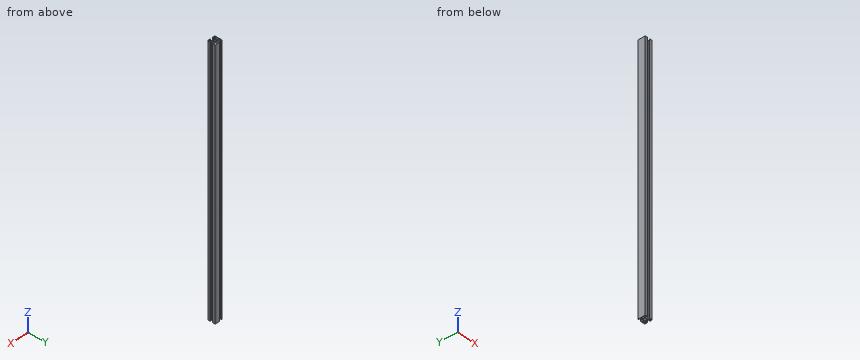
from build123d import *

# Parameters (mm, degrees)
SKETCH_1_R      = 2.25
EXTRUDE_1_DEPTH = 1000


with BuildPart() as part:
    # 草图1 → 拉伸1 (new body)
    with BuildSketch(Plane.XY):
        with BuildLine():
            Line((94.498219996, 123.603787887), (95.498219996, 123.603787887))
            Line((95.498219996, 123.603787887), (95.498219996, 120.604545229))
            Line((95.498219996, 120.604545229), (111.7555793, 120.604545229))
            ThreePointArc((111.7555793, 120.604545229), (112.138262733, 120.680665697), (112.462686082, 120.897438448))
            Line((112.462686082, 120.897438448), (114.705326774, 123.140079141))
            ThreePointArc((114.705326774, 123.140079141), (114.922099526, 123.46450249), (114.998219993, 123.847185922))
            Line((114.998219993, 123.847185922), (114.998219993, 125.604545228))
            ThreePointArc((114.998219993, 125.604545228), (114.705326774, 126.311652009), (113.998219993, 126.604545228))
            Line((113.998219993, 126.604545228), (104.998159012, 126.604545228))
            Line((104.998159012, 126.604545228), (104.998159012, 128.104545228))
            ThreePointArc((104.998159012, 128.104545228), (105.144605621, 128.458098618), (105.498159012, 128.604545228))
            Line((105.498159012, 128.604545228), (120.998159011, 128.604545228))
            ThreePointArc((120.998159011, 128.604545228), (122.412372573, 128.01875879), (122.998159011, 126.604545228))
            Line((122.998159011, 126.604545228), (122.998159011, 118.504545232))
            Line((122.998159011, 118.504545232), (122.198159011, 118.504545232))
            Line((122.198159011, 118.504545232), (122.198159011, 117.704545232))
            Line((122.198159011, 117.704545232), (120.798219991, 117.704545232))
            Line((120.798219991, 117.704545232), (120.798219991, 120.604545232))
            ThreePointArc((120.798219991, 120.604545232), (120.505326773, 121.311652013), (119.798219991, 121.604545232))
            Line((119.798219991, 121.604545232), (117.826647118, 121.604545232))
            ThreePointArc((117.826647118, 121.604545232), (117.443963686, 121.528424765), (117.119540337, 121.311652013))
            Line((117.119540337, 121.311652013), (115.291113212, 119.483224889))
            ThreePointArc((115.291113212, 119.483224889), (115.074340461, 119.15880154), (114.998219993, 118.776118107))
            Line((114.998219993, 118.776118107), (114.998219993, 108.432972357))
            ThreePointArc((114.998219993, 108.432972357), (115.074340461, 108.050288925), (115.291113212, 107.725865576))
            Line((115.291113212, 107.725865576), (117.119540337, 105.897438451))
            ThreePointArc((117.119540337, 105.897438451), (117.443963686, 105.6806657), (117.826647118, 105.604545232))
            Line((117.826647118, 105.604545232), (119.798219991, 105.604545232))
            ThreePointArc((119.798219991, 105.604545232), (120.505326773, 105.897438451), (120.798219991, 106.604545232))
            Line((120.798219991, 106.604545232), (120.798219991, 109.504545225))
            Line((120.798219991, 109.504545225), (122.198159011, 109.504545225))
            Line((122.198159011, 109.504545225), (122.198159011, 108.704545225))
            Line((122.198159011, 108.704545225), (122.998159011, 108.704545225))
            Line((122.998159011, 108.704545225), (122.998159011, 100.60454523))
            ThreePointArc((122.998159011, 100.60454523), (122.412372573, 99.190331667), (120.998159011, 98.60454523))
            Line((120.998159011, 98.60454523), (112.898159016, 98.60454523))
            Line((112.898159016, 98.60454523), (112.898159016, 99.40454523))
            Line((112.898159016, 99.40454523), (112.098159016, 99.40454523))
            Line((112.098159016, 99.40454523), (112.098159016, 100.804545237))
            Line((112.098159016, 100.804545237), (114.998219996, 100.804545237))
            ThreePointArc((114.998219996, 100.804545237), (115.705326777, 101.097438456), (115.998219996, 101.804545237))
            Line((115.998219996, 101.804545237), (115.998219996, 103.77611811))
            ThreePointArc((115.998219996, 103.77611811), (115.922099529, 104.158801543), (115.705326777, 104.483224892))
            Line((115.705326777, 104.483224892), (113.876899653, 106.311652016))
            ThreePointArc((113.876899653, 106.311652016), (113.552476304, 106.528424768), (113.169792871, 106.604545235))
            Line((113.169792871, 106.604545235), (102.826647121, 106.604545235))
            ThreePointArc((102.826647121, 106.604545235), (102.443963688, 106.528424768), (102.11954034, 106.311652016))
            Line((102.11954034, 106.311652016), (100.291113215, 104.483224892))
            ThreePointArc((100.291113215, 104.483224892), (100.074340464, 104.158801543), (99.998219996, 103.77611811))
            Line((99.998219996, 103.77611811), (99.998219996, 101.804545237))
            ThreePointArc((99.998219996, 101.804545237), (100.291113215, 101.097438456), (100.998219996, 100.804545237))
            Line((100.998219996, 100.804545237), (103.898159009, 100.804545237))
            Line((103.898159009, 100.804545237), (103.898159009, 99.40454523))
            Line((103.898159009, 99.40454523), (103.098159009, 99.40454523))
            Line((103.098159009, 99.40454523), (103.098159009, 98.60454523))
            Line((103.098159009, 98.60454523), (94.998159011, 98.60454523))
            ThreePointArc((94.998159011, 98.60454523), (93.583945449, 99.190331667), (92.998159011, 100.60454523))
            Line((92.998159011, 100.60454523), (92.998159011, 126.604545228))
            ThreePointArc((92.998159011, 126.604545228), (93.583945449, 128.01875879), (94.998159011, 128.604545228))
            Line((94.998159011, 128.604545228), (95.498219996, 128.604545228))
            Line((95.498219996, 128.604545228), (95.498219996, 125.603787887))
            Line((95.498219996, 125.603787887), (94.498219996, 125.603787887))
            Line((94.498219996, 125.603787887), (94.498219996, 123.603787887))
        make_face()
        with Locations((119.498219995, 102.104545233)):
            Circle(SKETCH_1_R, mode=Mode.SUBTRACT)
        with BuildLine():
            Line((97.998219996, 104.1812012), (97.998219996, 105.19033167))
            ThreePointArc((97.998219996, 105.19033167), (98.074340464, 105.573015102), (98.291113215, 105.897438451))
            Line((98.291113215, 105.897438451), (100.70532678, 108.311652016))
            ThreePointArc((100.70532678, 108.311652016), (100.922099531, 108.636075365), (100.998219999, 109.018758797))
            Line((100.998219999, 109.018758797), (100.998219999, 117.604545229))
            ThreePointArc((100.998219999, 117.604545229), (100.70532678, 118.311652011), (99.998219999, 118.604545229))
            Line((99.998219999, 118.604545229), (95.198219996, 118.604545229))
            Line((95.198219996, 118.604545229), (95.198219996, 104.400737733))
            ThreePointArc((95.198219996, 104.400737733), (95.122257957, 104.018437006), (94.905912304, 103.694216964))
            ThreePointArc((94.905912304, 103.694216964), (96.395419712, 99.856894882), (98.228989227, 103.542230133))
            ThreePointArc((98.228989227, 103.542230133), (98.057680053, 103.841518089), (97.998219996, 104.1812012))
        make_face(mode=Mode.SUBTRACT)
        with BuildLine():
            ThreePointArc((103.573125257, 115.932320253), (102.998219996, 113.604545232), (103.573125257, 111.276770211))
            ThreePointArc((103.573125257, 111.276770211), (103.402025918, 109.008351155), (105.670444975, 109.179450493))
            ThreePointArc((105.670444975, 109.179450493), (107.998219996, 108.604545232), (110.325995017, 109.179450493))
            ThreePointArc((110.325995017, 109.179450493), (112.594414074, 109.008351155), (112.423314735, 111.276770211))
            ThreePointArc((112.423314735, 111.276770211), (112.998219996, 113.604545232), (112.423314735, 115.932320253))
            ThreePointArc((112.423314735, 115.932320253), (112.594414074, 118.20073931), (110.325995017, 118.029639971))
            ThreePointArc((110.325995017, 118.029639971), (107.998219996, 118.604545232), (105.670444975, 118.029639971))
            ThreePointArc((105.670444975, 118.029639971), (103.402025918, 118.20073931), (103.573125257, 115.932320253))
        make_face(mode=Mode.SUBTRACT)
    extrude(amount=EXTRUDE_1_DEPTH)


solid = part.part
Geometry: final body of the model. Coordinates: model frame, mm. Round coordinates to 2 decimals unless told otherwise and drop trailing zeros.
Q1. Section A-A, the plane z = 601. Give the number of separate pieces and of enclosed holes in the cut face, and give its area (3 significant figures).
Result sheet:
separate pieces: 1
enclosed holes: 3
area: 351 mm2
Q2. Material intervals for probe 1 along X at (y, z) = (109.25, 392.5); probe 2 along X at (y, z) = (110.5, 182); probe 3 along X at (y, z) = (105, 646.5), sorted ascending.
Result sheet:
probe 1: x = 93 to 95.2, 101 to 103.21, 112.79 to 115, 120.8 to 122.2
probe 2: x = 93 to 95.2, 101 to 103.03, 112.97 to 115
probe 3: x = 93 to 95.2, 98 to 100.81, 115.19 to 123
Q3. Pin query (flat end, axial travel): pin 1 (0.9 mm diameter, centred on y = 99, z = 548, fed in from +X); pin 2 (5 mm diameter, centred on x = 106, z = 462, fed in from -Y); pin 3 (1 mm diameter, centred on y = 109.5, z = 480.5, fed in from +X). Return the tip coordinate at first contact, or that it passes through.
Result sheet:
pin 1: stops at x = 122.63
pin 2: stops at y = 99.4
pin 3: stops at x = 122.2
